Geometry check sheet. Reference: drawing and pictorial views, mm from the part's lowest x, y, z. A direction names the side the tool comes from. Give positions to 0.01 mm unless a question says otherwise; leave off trailing zeros. Loops run counter-clockwise (first coordinate to the right, second up) from the corner with the lowest first, then second, coordinate; pieces in that order, holes last. Notation, with made-up numbers: (-40, 36) - (-34, 36) arc R12 cw to (-34, 47) - close; hole circle Ø1 at (-10.5, 0.5). An arc over 180 degrees is marked (long way). One line per question, with ' | ' between items. Start each with the question number.
1. Mould release check, pull along X, two halves, no side actions. Record for the marked faces 4, 5 and 6: +X half, -X half, draft (parallel to the pull), parting line (faces both ways), or undercut.
2. Section check B-B, the plane y = 4.75. Enter the section's corners in (x, z).
3. Section check D-D, the plane z = 2.35. Enter the section's corners in (x, y).
4. Thickness scan on line 1 along X through (y, z) = (5.5, 0.9); line 2 along Z through (x, y) = (8, 4.75); line 3 along X through (y, z) = (5.25, 1.55) (1 decimal). Record the ranges inside material, lowest first. Write a range as from..to.
5. Tool access check on the marked faces 1, 2 and 3. Record the directions out of +Z, -Z, +X, -X, +Y, -Y that give a thin tool (end or side, any length) a straight path to the whole face; none if there is none.
6. Depth check by flat-ended pin: pin 1 Ø0.5 at (y, z) = (6, 0.5) entering from +X; pin 2 Ø1.1 at (y, z) = (3, 0.5) entering from +X; pin 3 Ø0.8 at (y, z) = (6.5, 0.5) entering from -X. Enter the tip coordinate at first touch or a pass-through.
7. Section check C-C, the plane x = 4.75. Enter the section's corners in (y, z).
8. Section check A-A, the plane z = 0.55. Enter the section's corners in (x, y).
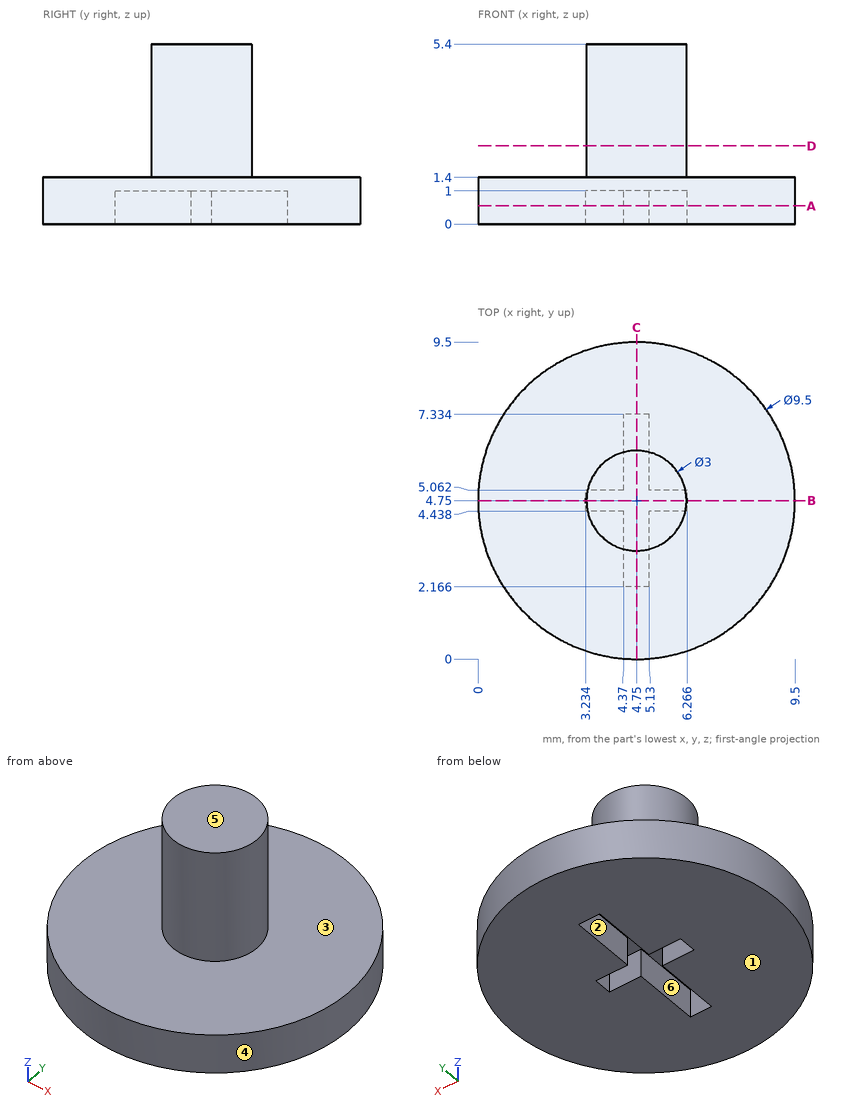
Results list:
1) face 4: parting line | face 5: draft | face 6: undercut
2) outline: (0, 0) - (3.23, 0) - (3.23, 1) - (6.27, 1) - (6.27, 0) - (9.5, 0) - (9.5, 1.4) - (6.25, 1.4) - (6.25, 5.4) - (3.25, 5.4) - (3.25, 1.4) - (0, 1.4) - close
3) outline: circle Ø3 at (4.75, 4.75)
4) line 1: 0.06..4.37, 5.13..9.44 | line 2: 0..1.4 | line 3: 3.3..6.2
5) face 1: -Z, +X, -X, +Y, -Y | face 2: -Z | face 3: +Z
6) pin 1: x = 9.39 | pin 2: x = 9.35 | pin 3: x = 0.2
7) outline: (0, 0) - (2.17, 0) - (2.17, 1) - (7.33, 1) - (7.33, 0) - (9.5, 0) - (9.5, 1.4) - (6.25, 1.4) - (6.25, 5.4) - (3.25, 5.4) - (3.25, 1.4) - (0, 1.4) - close
8) outline: circle Ø9.5 at (4.75, 4.75); hole (3.23, 4.44) - (4.37, 4.44) - (4.37, 2.17) - (5.13, 2.17) - (5.13, 4.44) - (6.27, 4.44) - (6.27, 5.06) - (5.13, 5.06) - (5.13, 7.33) - (4.37, 7.33) - (4.37, 5.06) - (3.23, 5.06) - close
